from build123d import *

# Parameters (mm, degrees)
SKETCH1_W           = 45
SKETCH1_H           = 20
SKETCH1_H_2         = 68.5
SKETCH1_W_2         = 9
SKETCH1_W_3         = 23.5
SKETCH1_H_3         = 23.5
BOSS_EXTRUDE1_DEPTH = 2
SKETCH1_3_W         = 23.5
SKETCH1_3_H         = 23.5
SKETCH1_3_W_2       = 45
SKETCH1_3_H_2       = 20
BOSS_EXTRUDE2_DEPTH = 12


with BuildPart() as part:
    # Sketch1 → Boss-Extrude1 (new body)
    # profile 1 of 11: a face of its own
    with BuildSketch(Plane(origin=(0, 0, 0), x_dir=(1, 0, 0), z_dir=(0, 1, 0))):
        Polygon((0, 92.1), (0, 0), (221.7, 0), (221.7, 92.1), (219.9, 92.1), (219.9, 23.6), (174.9, 23.6), (174.9, 92.1), (173.9, 92.1), (173.9, 23.6), (164.9, 23.6), (164.9, 92.1), (163.9, 92.1), (163.9, 23.6), (118.9, 23.6), (118.9, 92.1), (117.1, 92.1), (117.1, 23.6), (72.1, 23.6), (72.1, 92.1), (70.3, 92.1), (70.3, 23.6), (1.8, 23.6), (1.8, 68.6), (1.8, 92.1), align=None)
        with Locations((47.8, 11.8)):
            Rectangle(SKETCH1_W, SKETCH1_H, mode=Mode.SUBTRACT)
        with Locations((94.6, 11.8)):
            Rectangle(SKETCH1_W, SKETCH1_H, mode=Mode.SUBTRACT)
        with Locations((141.4, 11.8)):
            Rectangle(SKETCH1_W, SKETCH1_H, mode=Mode.SUBTRACT)
        with Locations((197.4, 11.8)):
            Rectangle(SKETCH1_W, SKETCH1_H, mode=Mode.SUBTRACT)
    # profile 2 of 11: a face of its own
    with BuildSketch(Plane(origin=(0, 0, 0), x_dir=(1, 0, 0), z_dir=(0, 1, 0))):
        with Locations((47.8, 11.8)):
            Rectangle(SKETCH1_W, SKETCH1_H)
    # profile 3 of 11: a face of its own
    with BuildSketch(Plane(origin=(0, 0, 0), x_dir=(1, 0, 0), z_dir=(0, 1, 0))):
        Polygon((70.3, 92.1), (25.3, 92.1), (25.3, 68.6), (1.8, 68.6), (1.8, 23.6), (70.3, 23.6), align=None)
    # profile 4 of 11: a face of its own
    with BuildSketch(Plane(origin=(0, 0, 0), x_dir=(1, 0, 0), z_dir=(0, 1, 0))):
        with Locations((94.6, 57.85)):
            Rectangle(SKETCH1_W, SKETCH1_H_2)
    # profile 5 of 11: a face of its own
    with BuildSketch(Plane(origin=(0, 0, 0), x_dir=(1, 0, 0), z_dir=(0, 1, 0))):
        with Locations((94.6, 11.8)):
            Rectangle(SKETCH1_W, SKETCH1_H)
    # profile 6 of 11: a face of its own
    with BuildSketch(Plane(origin=(0, 0, 0), x_dir=(1, 0, 0), z_dir=(0, 1, 0))):
        with Locations((141.4, 11.8)):
            Rectangle(SKETCH1_W, SKETCH1_H)
    # profile 7 of 11: a face of its own
    with BuildSketch(Plane(origin=(0, 0, 0), x_dir=(1, 0, 0), z_dir=(0, 1, 0))):
        with Locations((141.4, 57.85)):
            Rectangle(SKETCH1_W, SKETCH1_H_2)
    # profile 8 of 11: a face of its own
    with BuildSketch(Plane(origin=(0, 0, 0), x_dir=(1, 0, 0), z_dir=(0, 1, 0))):
        with Locations((197.4, 11.8)):
            Rectangle(SKETCH1_W, SKETCH1_H)
    # profile 9 of 11: a face of its own
    with BuildSketch(Plane(origin=(0, 0, 0), x_dir=(1, 0, 0), z_dir=(0, 1, 0))):
        with Locations((197.4, 57.85)):
            Rectangle(SKETCH1_W, SKETCH1_H_2)
    # profile 10 of 11: a face of its own
    with BuildSketch(Plane(origin=(0, 0, 0), x_dir=(1, 0, 0), z_dir=(0, 1, 0))):
        with Locations((169.4, 57.85)):
            Rectangle(SKETCH1_W_2, SKETCH1_H_2)
    # profile 11 of 11: a face of its own
    with BuildSketch(Plane(origin=(0, 0, 0), x_dir=(1, 0, 0), z_dir=(0, 1, 0))):
        with Locations((13.55, 80.35)):
            Rectangle(SKETCH1_W_3, SKETCH1_H_3)
    extrude(amount=-BOSS_EXTRUDE1_DEPTH)

    # Sketch1_3 → Boss-Extrude2 (add)
    # profile 1 of 2: a face of its own
    with BuildSketch(Plane(origin=(0, 0, 0), x_dir=(1, 0, 0), z_dir=(0, 1, 0))):
        with Locations((13.55, 80.35)):
            Rectangle(SKETCH1_3_W, SKETCH1_3_H)
    # profile 2 of 2: a face of its own
    with BuildSketch(Plane(origin=(0, 0, 0), x_dir=(1, 0, 0), z_dir=(0, 1, 0))):
        Polygon((0, 92.1), (0, 0), (221.7, 0), (221.7, 92.1), (219.9, 92.1), (219.9, 23.6), (174.9, 23.6), (174.9, 92.1), (173.9, 92.1), (173.9, 23.6), (164.9, 23.6), (164.9, 92.1), (163.9, 92.1), (163.9, 23.6), (118.9, 23.6), (118.9, 92.1), (117.1, 92.1), (117.1, 23.6), (72.1, 23.6), (72.1, 92.1), (70.3, 92.1), (70.3, 23.6), (1.8, 23.6), (1.8, 68.6), (1.8, 92.1), align=None)
        with Locations((47.8, 11.8)):
            Rectangle(SKETCH1_3_W_2, SKETCH1_3_H_2, mode=Mode.SUBTRACT)
        with Locations((94.6, 11.8)):
            Rectangle(SKETCH1_3_W_2, SKETCH1_3_H_2, mode=Mode.SUBTRACT)
        with Locations((141.4, 11.8)):
            Rectangle(SKETCH1_3_W_2, SKETCH1_3_H_2, mode=Mode.SUBTRACT)
        with Locations((197.4, 11.8)):
            Rectangle(SKETCH1_3_W_2, SKETCH1_3_H_2, mode=Mode.SUBTRACT)
    extrude(amount=BOSS_EXTRUDE2_DEPTH)


solid = part.part
Work out the finished part from the listing and answer in its coordinate system (mm). A direction names the side the tool comes from. Round coordinates to 2 decimals unless told otherwise and drop trailing zeros. Loops run counter-clockwise (first coordinate to the right, second up) from the corner with the lowest first, then second, coordinate; pieces in that order, holes last. Notation, with made-up numbers: (-24, 74.25) -> (21, 74.25) arc R18 cw to (21, 89.25) -> close; hole circle Ø5 at (6.25, -7.5). An arc over 180 degrees is marked (long way). Use one line per item in the form item = value.
(1) Find section A-A on x = 125. Give the vertices of the cut face in (y, z), then the cut area to 3 significant figures.
Answer list:
outline = (-2, -92.1) -> (0, -92.1) -> (0, -23.6) -> (12, -23.6) -> (12, -21.8) -> (0, -21.8) -> (0, -1.8) -> (12, -1.8) -> (12, 0) -> (-2, 0) -> close
area = 227 mm2
(2) Find section B-B on z = -80. Give the vertices of the cut face in (x, y).
Answer list:
outline = (0, -2) -> (221.7, -2) -> (221.7, 12) -> (219.9, 12) -> (219.9, 0) -> (174.9, 0) -> (174.9, 12) -> (173.9, 12) -> (173.9, 0) -> (164.9, 0) -> (164.9, 12) -> (163.9, 12) -> (163.9, 0) -> (118.9, 0) -> (118.9, 12) -> (117.1, 12) -> (117.1, 0) -> (72.1, 0) -> (72.1, 12) -> (70.3, 12) -> (70.3, 0) -> (25.3, 0) -> (25.3, 12) -> (0, 12) -> close
(3) Flat-ended cylindrical pins translate along their axes: P1, Ø6, axis at x = 135.5, y = 7, coming from the -Z side; P2, Ø22.5, axis at x = 101, z = -50, coming from the +Y side; P3, Ø6, axis at y = 4.5, z = -11.5, coming from the -X side. Find the tip coordinate at first contact, or state that the pin passes through.
Answer list:
P1 = -23.6
P2 = 0
P3 = 0
(4) A tool of negligible diameter and unlimited length cuts with its end or side. For faces 4 (the flat face through (0, 5, -47)), 5 (the flat face through (219.9, 6, -58)), 6 (the flat face through (118.9, 6, -12)), from which of +Z, -Z, +X, -X, +Y, -Y can it reach the whole face along a straight path? Write none if from no direction.
Answer list:
face_4 = +Z, -Z, -X, +Y, -Y
face_5 = -Z, +Y
face_6 = +Y
(5) For a pull along Z with two mould halves and no side action, classify faces 1 (the flat face through (109, 5, 0)), 2 (the flat face through (72.1, 6, -57)), 3 (the flat face through (94, 6, -21.8)) as released by +Z, released by -Z, zero draft, split by the parting line, or undercut.
Answer list:
face_1 = released by +Z
face_2 = zero draft
face_3 = undercut
(6) Find section C-C on y = 3.25. Give the number of separate pieces and of enclosed holes in the cut face, then the cut area to 3 significant figures.
Answer list:
separate_pieces = 1
enclosed_holes = 4
area = 2,810 mm2
(7) Find section D-D on z = -65.5. Give the vertices of the cut face in (x, y), then the cut area to 3 significant figures.
Answer list:
outline = (0, -2) -> (221.7, -2) -> (221.7, 12) -> (219.9, 12) -> (219.9, 0) -> (174.9, 0) -> (174.9, 12) -> (173.9, 12) -> (173.9, 0) -> (164.9, 0) -> (164.9, 12) -> (163.9, 12) -> (163.9, 0) -> (118.9, 0) -> (118.9, 12) -> (117.1, 12) -> (117.1, 0) -> (72.1, 0) -> (72.1, 12) -> (70.3, 12) -> (70.3, 0) -> (1.8, 0) -> (1.8, 12) -> (0, 12) -> close
area = 554 mm2
(8) Straight lines are drawn through the part: line 1 (X direction, y = 2, z = -9.5); line 2 (X direction, y = 8.5, z = -25); line 3 (Z direction, x = 89, y = 3). For each, find the intervals that lie inside material, in ascending order.
Answer list:
line_1 = 0 to 25.3, 70.3 to 72.1, 117.1 to 118.9, 163.9 to 174.9, 219.9 to 221.7
line_2 = 0 to 1.8, 70.3 to 72.1, 117.1 to 118.9, 163.9 to 164.9, 173.9 to 174.9, 219.9 to 221.7
line_3 = -23.6 to -21.8, -1.8 to 0
